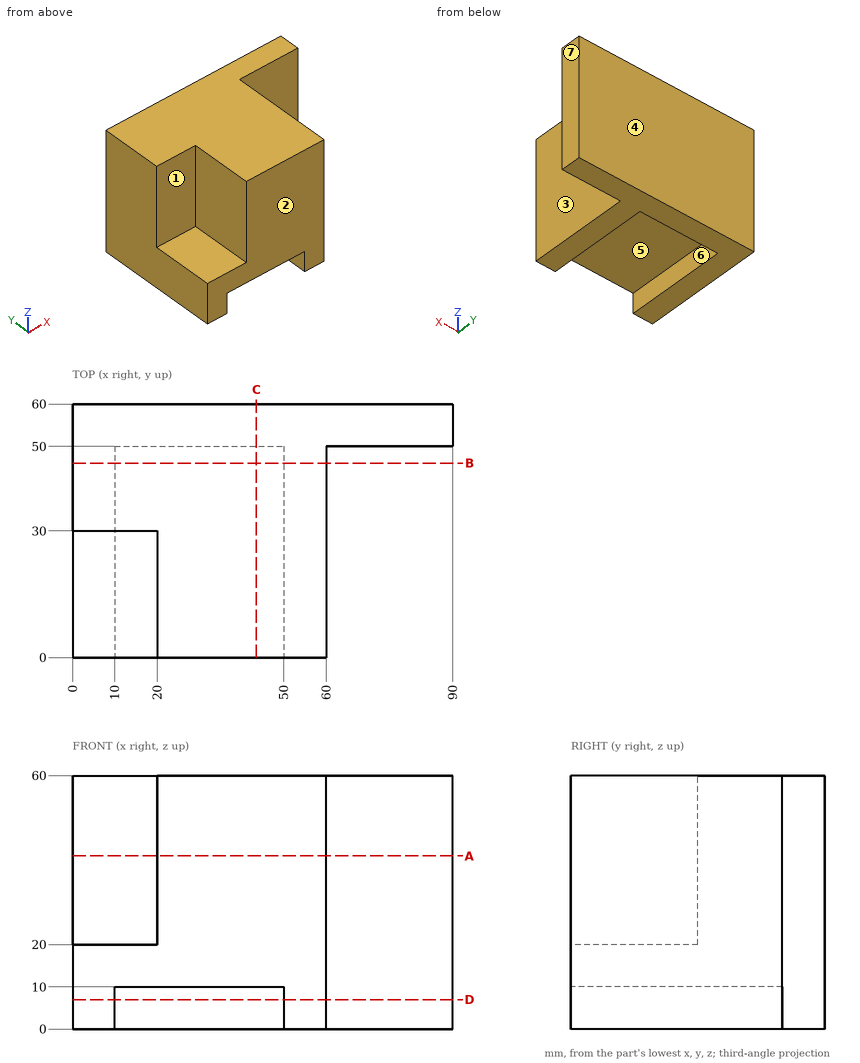
The drawing under review shows one solid part. Ordinate dimensions are in mm from its lowest x, y, z. A direction names the side the tool comes from. Round coordinates to 2 decimals unless told otherwise and drop trailing zeros. Loops run counter-clockwise (first coordinate to the right, second up) from the corner with the lowest first, then second, coordinate; pieces in that order, holes last. Notation, with made-up numbers: (10, -15.5) - (43, -15.5) arc R31 cw to (43, 18.5) - close; hole circle Ø10 at (-21.5, 77.5). An arc over 180 degrees is marked (long way). Put each result on its own line as item: value. Start each with the question number.
1. For probe 1 along X at (y, z) = (15, 3); probe 2 along X at (y, z) = (22.5, 30); probe 3 along Z at (x, y) = (12, 4.5), list the stretches that pass through material, from the lowest coordinate up. Write a range as [from, to].
2. Insertion check: P1, Ø1.5, axis at x = 44.5, y = 43, coming from the -Z side; P2, Ø6, axis at x = 14, y = 7.5, coming from the +Z side; P3, Ø1, axis at y = 6, z = 38.5, coming from the +X side. Each pin has a flat end and moves straight along its axis. Give the tip position at first contact, or say it passes through.
3. For the marked faces 1, 2 and 3, list the 3-axis set-ups (+Z, -Z, +X, -X, +Y, -Y) from which the entire face can be reached by the end or side of a thin tool; tool diameter is ignored.
4. Mouldability with a two-part tool opening along X and no side actions: class the marked faces 4, 5, 6 and 7 as +X half, -X half, draft (parallel to the pull), parting line (faces both ways), or undercut.
5. Consider section A-A on z = 41. State the section outline as (x, y) points, plus the area to 3 significant figures.
6. Consider section D-D on z = 7. State the section outline as (x, y) points, plus the area to 3 significant figures.
7. Consider section C-C on x = 43.5. State the section outline as (y, z) points, plus the area to 3 significant figures.
8. Consider section B-B on y = 46. State the section outline as (x, z) points, plus the area to 3 significant figures.
Result sheet:
1. probe 1: [0, 10], [50, 60]
1. probe 2: [20, 60]
1. probe 3: [10, 20]
2. P1: z = 10
2. P2: z = 20
2. P3: x = 60
3. face 1: +Z, -X, -Y
3. face 2: +Z, -Z, +X, -X, -Y
3. face 3: +Z, -Z, +X, -Y
4. face 4: draft
4. face 5: undercut
4. face 6: undercut
4. face 7: +X half
5. outline: (0, 30) - (20, 30) - (20, 0) - (60, 0) - (60, 50) - (90, 50) - (90, 60) - (0, 60) - close
5. area: 3,300 mm^2
6. outline: (0, 0) - (10, 0) - (10, 50) - (50, 50) - (50, 0) - (60, 0) - (60, 50) - (90, 50) - (90, 60) - (0, 60) - close
6. area: 1,900 mm^2
7. outline: (0, 10) - (50, 10) - (50, 0) - (60, 0) - (60, 60) - (0, 60) - close
7. area: 3,100 mm^2
8. outline: (0, 0) - (10, 0) - (10, 10) - (50, 10) - (50, 0) - (60, 0) - (60, 60) - (0, 60) - close
8. area: 3,200 mm^2
